The listing builds one solid part. Answer for the finished solid, in the listing's coordinates (mm). Coordinates: 2 decimals unless noted, no trailing zeros. Loops run counter-clockwise (first coordinate to the right, second up) from the corner with the lowest first, then second, coordinate; pieces in that order, holes last. Notation, with made-up numbers: (18.25, -6) -> (70.25, -6) arc R8 ccw to (70.25, 8) -> close; hole circle Ø4 at (20, 61.25). An arc over 180 degrees is marked (long way). Answer in a Markdown table with one row per item.
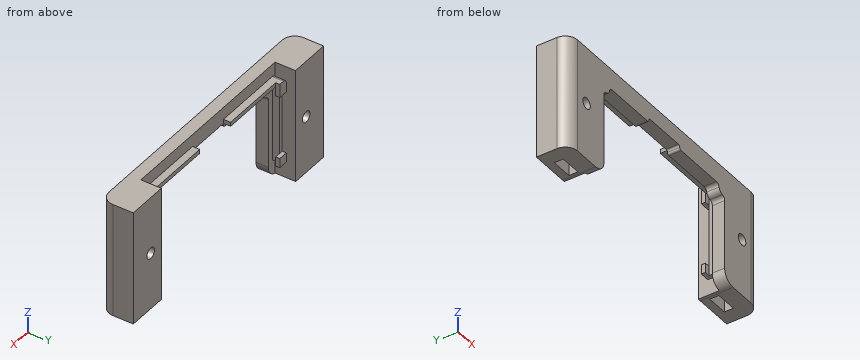
```python
from build123d import *

# Parameters (mm, degrees)
SKETCH1_R                = 8.05
SKETCH1_R_2              = 0.8
BOSS_EXTRUDE1_DEPTH      = 3
SKETCH1_5_R              = 0.8
BOSS_EXTRUDE3_DEPTH      = 3
CUT_EXTRUDE2_REACH       = 32.121
SKETCH5_R                = 8.05
FILLET2_R                = 1
BOSS_EXTRUDE4_DEPTH      = 1.75
BOSS_EXTRUDE7_START      = 1.75
SKETCH6_5_W              = 2.32
SKETCH6_5_H              = 2.32
BOSS_EXTRUDE7_DEPTH      = 1
SKETCH7_W                = 10
SKETCH7_H                = 28
BOSS_EXTRUDE8_DEPTH      = 8
SKETCH8_R                = 1.35
CUT_EXTRUDE3_DEPTH       = 1.1
CUT_EXTRUDE4_DEPTH       = 38.01634774
CUT_EXTRUDE4_DEPTH_BACK  = 38.01634774
SKETCH8_3_R              = 1.35
BOSS_EXTRUDE9_DEPTH      = 20
BOSS_EXTRUDE9_DEPTH_BACK = 20
SKETCH10_W               = 5
SKETCH10_H               = 3
CUT_EXTRUDE5_REACH       = 39.539
SKETCH9_W                = 43
SKETCH9_H                = 7.971706725
CUT_EXTRUDE6_REACH       = 39.016
SKETCH12_W               = 11
SKETCH12_H               = 1
FILLET3_R                = 3
FILLET4_START            = -1
FILLET4_DEPTH            = 5
FILLET4_2_DEPTH          = 3


with BuildPart() as part:
    # Sketch1 → Boss-Extrude1 (new body)
    with BuildSketch(Plane(origin=(0, 0, 0), x_dir=(1, 0, 0), z_dir=(0, 1, 0))):
        with BuildLine():
            Line((5.5, -7), (5.5, -14))
            Line((5.5, -14), (25.5, -14))
            ThreePointArc((25.5, -14), (26.207106781, -13.707106781), (26.5, -13))
            Line((26.5, -13), (26.5, 13))
            ThreePointArc((26.5, 13), (26.207106781, 13.707106781), (25.5, 14))
            Line((25.5, 14), (-25.5, 14))
            ThreePointArc((-25.5, 14), (-26.207106781, 13.707106781), (-26.5, 13))
            Line((-26.5, 13), (-26.5, -13))
            ThreePointArc((-26.5, -13), (-26.207106781, -13.707106781), (-25.5, -14))
            Line((-25.5, -14), (-5.5, -14))
            Line((-5.5, -14), (-5.5, -7))
            Line((-5.5, -7), (5.5, -7))
        make_face()
        with Locations(Location((-12.95, 0, 0), (0, 0, 270))):
            Circle(SKETCH1_R, mode=Mode.SUBTRACT)
        with Locations(Location((12.95, 0, 0), (0, 0, 270))):
            Circle(SKETCH1_R, mode=Mode.SUBTRACT)
        with BuildLine():
            ThreePointArc((-3.25, 5.75), (-5.25, 7.75), (-3.25, 9.75))
            Line((-3.25, 9.75), (3.25, 9.75))
            ThreePointArc((3.25, 9.75), (5.25, 7.75), (3.25, 5.75))
            Line((3.25, 5.75), (-3.25, 5.75))
        make_face(mode=Mode.SUBTRACT)
        with Locations(Location((-20.99, 8.49, 0), (0, 0, 270))):
            Circle(SKETCH1_R_2, mode=Mode.SUBTRACT)
        with Locations(Location((20.99, 8.49, 0), (0, 0, 270))):
            Circle(SKETCH1_R_2, mode=Mode.SUBTRACT)
        with Locations(Location((20.99, -8.49, 0), (0, 0, 270))):
            Circle(SKETCH1_R_2, mode=Mode.SUBTRACT)
        with Locations(Location((-20.99, -8.49, 0), (0, 0, 270))):
            Circle(SKETCH1_R_2, mode=Mode.SUBTRACT)
    extrude(amount=BOSS_EXTRUDE1_DEPTH)

    # Sketch1<5> → Boss-Extrude3 (add)
    with BuildSketch(Plane(origin=(0, 0, 0), x_dir=(1, 0, 0), z_dir=(0, 1, 0))):
        with Locations((20.99, 8.49)):
            Circle(SKETCH1_5_R)
        with Locations((-20.99, 8.49)):
            Circle(SKETCH1_5_R)
        with Locations((-20.99, -8.49)):
            Circle(SKETCH1_5_R)
        with Locations((20.99, -8.49)):
            Circle(SKETCH1_5_R)
    extrude(amount=BOSS_EXTRUDE3_DEPTH)

    # Sketch5 → Cut-Extrude2 (cut, up to next)
    with BuildSketch(Plane(origin=(0, 3, 0), x_dir=(1, 0, 0), z_dir=(0, 1, 0)), mode=Mode.PRIVATE) as cut_extrude2_sk1:
        with BuildLine():
            Line((3.25, 5.75), (-3.25, 5.75))
            ThreePointArc((-3.25, 5.75), (-5.052775638, 6.883974596), (-4.8112495, 9))
            Line((-4.8112495, 9), (-19.56873296, 9))
            ThreePointArc((-19.56873296, 9), (-19.502348624, 8.748830803), (-19.48, 8.49))
            ThreePointArc((-19.48, 8.49), (-20.12109264, 7.255050608), (-21.5, 7.06873296))
            Line((-21.5, 7.06873296), (-21.5, -7.06873296))
            ThreePointArc((-21.5, -7.06873296), (-20.12109264, -7.255050608), (-19.48, -8.49))
            ThreePointArc((-19.48, -8.49), (-19.502348624, -8.748830803), (-19.56873296, -9))
            Line((-19.56873296, -9), (-5.5, -9))
            Line((-5.5, -9), (-5.5, -7))
            Line((-5.5, -7), (5.5, -7))
            Line((5.5, -7), (5.5, -9))
            Line((5.5, -9), (19.56873296, -9))
            ThreePointArc((19.56873296, -9), (19.92226876, -7.42226876), (21.5, -7.06873296))
            Line((21.5, -7.06873296), (21.5, 7.06873296))
            ThreePointArc((21.5, 7.06873296), (19.92226876, 7.42226876), (19.56873296, 9))
            Line((19.56873296, 9), (4.8112495, 9))
            ThreePointArc((4.8112495, 9), (5.052775638, 6.883974596), (3.25, 5.75))
        make_face()
        with Locations((-12.95, 0)):
            Circle(SKETCH5_R, mode=Mode.SUBTRACT)
        with Locations((12.95, 0)):
            Circle(SKETCH5_R, mode=Mode.SUBTRACT)
    cut_extrude2_tool1 = extrude(cut_extrude2_sk1.sketch, amount=-CUT_EXTRUDE2_REACH, mode=Mode.PRIVATE) & part.part
    add(cut_extrude2_tool1.solids().sort_by_distance((0, 3, 0.207713))[0], mode=Mode.SUBTRACT)

    # Fillet2
    fillet2_edges = [part.edges().sort_by_distance(p)[0] for p in [
        (21.5, 1.5, 7.06873296),
        (19.56873296, 1.5, 9),
        (5.5, 1.5, 9),
        (-5.5, 1.5, 9),
        (-19.56873296, 1.5, 9),
        (-21.5, 1.5, 7.06873296),
        (-21.5, 1.5, -7.06873296),
        (-19.56873296, 1.5, -9),
        (-4.8112495, 1.5, -9),
        (4.8112495, 1.5, -9),
        (19.56873296, 1.5, -9),
        (21.5, 1.5, -7.06873296),
    ]]
    fillet(fillet2_edges, radius=FILLET2_R)

    # Sketch6 → Boss-Extrude4 (add)
    with BuildSketch(Plane(origin=(0, 3, 0), x_dir=(1, 0, 0), z_dir=(0, 1, 0))):
        with BuildLine():
            ThreePointArc((-23.9, -10), (-23.607106781, -10.707106781), (-22.9, -11))
            Line((-22.9, -11), (-5.5, -11))
            Line((-5.5, -11), (-5.5, -10))
            Line((-5.5, -10), (-22.9, -10))
            Line((-22.9, -10), (-22.9, 10))
            Line((-22.9, 10), (-23.9, 10))
            Line((-23.9, 10), (-23.9, -10))
        make_face()
    boss_extrude4 = extrude(amount=BOSS_EXTRUDE4_DEPTH)

    # Sketch6<5> → Boss-Extrude7 (add)
    with BuildSketch(Plane(origin=(0, 3, 0), x_dir=(1, 0, 0), z_dir=(0, 1, 0)).offset(BOSS_EXTRUDE7_START)):
        with BuildLine():
            Line((-23.9, -7.68), (-23.9, -10))
            ThreePointArc((-23.9, -10), (-23.607106781, -10.707106781), (-22.9, -11))
            Line((-22.9, -11), (-21.58, -11))
            Line((-21.58, -11), (-21.58, -7.68))
            Line((-21.58, -7.68), (-23.9, -7.68))
        make_face()
        with Locations((-22.74, 8.84)):
            Rectangle(SKETCH6_5_W, SKETCH6_5_H)
    boss_extrude7 = extrude(amount=BOSS_EXTRUDE7_DEPTH)

    # Mirror1: Boss-Extrude4, Boss-Extrude7 across plane
    add(boss_extrude4.mirror(Plane(origin=(0, 0, 0), x_dir=(0, 0, 1), z_dir=(1, 0, 0))))
    add(boss_extrude7.mirror(Plane(origin=(0, 0, 0), x_dir=(0, 0, 1), z_dir=(1, 0, 0))))

    # Sketch7 → Boss-Extrude8 (add)
    with BuildSketch(Plane(origin=(0, 0, 0), x_dir=(1, 0, 0), z_dir=(0, 1, 0))):
        with Locations((-28.9, 0)):
            Rectangle(SKETCH7_W, SKETCH7_H)
        with Locations((28.9, 0)):
            Rectangle(SKETCH7_W, SKETCH7_H)
    extrude(amount=BOSS_EXTRUDE8_DEPTH)

    # Sketch8 → Cut-Extrude3 (cut, symmetric)
    with BuildSketch(Plane(origin=(0, 5, 0), x_dir=(-1, 0, 0), z_dir=(0, -1, 0))):
        Polygon((-30.3, 1.5011107), (-30.3, -1.5011107), (-27.7, -3.0022214), (-25.1, -1.5011107), (-25.1, 1.5011107), (-27.7, 3.0022214), align=None)
        Polygon((-25.1, 1.5011107), (-25.1, 14), (-30.3, 14), (-30.3, 1.5011107), (-27.7, 3.0022214), align=None)
        Polygon((25.1, 14), (30.3, 14), (30.3, 1.5011107), (27.7, 3.0022214), (25.1, 1.5011107), align=None)
        Polygon((30.3, -1.5011107), (27.7, -3.0022214), (25.1, -1.5011107), (25.1, 1.5011107), (27.7, 3.0022214), (30.3, 1.5011107), align=None)
        with Locations((27.7, 0)):
            Circle(SKETCH8_R)
        with Locations((-27.7, 0)):
            Circle(SKETCH8_R)
    extrude(amount=CUT_EXTRUDE3_DEPTH, both=True, mode=Mode.SUBTRACT)

    # Sketch8<3> → Cut-Extrude4 (cut, two sides: drawn at the far end of the back side and taken through both)
    with BuildSketch(Plane(origin=(0, 5, 0), x_dir=(-1, 0, 0), z_dir=(0, -1, 0)).offset(-CUT_EXTRUDE4_DEPTH_BACK)):
        with Locations(Location((-27.7, 0, 0), (0, 0, 90))):
            Circle(SKETCH8_3_R)
        with Locations(Location((27.7, 0, 0), (0, 0, 90))):
            Circle(SKETCH8_3_R)
    extrude(amount=CUT_EXTRUDE4_DEPTH + CUT_EXTRUDE4_DEPTH_BACK, mode=Mode.SUBTRACT)

    # Sketch10 → Boss-Extrude9 (add, two sides: drawn at the far end of the back side and taken through both)
    with BuildSketch(Plane(origin=(-5.5, 0, 0), x_dir=(0, 0, -1), z_dir=(1, 0, 0)).offset(-BOSS_EXTRUDE9_DEPTH_BACK)):
        with Locations((-11.5, 1.5)):
            Rectangle(SKETCH10_W, SKETCH10_H)
    extrude(amount=BOSS_EXTRUDE9_DEPTH + BOSS_EXTRUDE9_DEPTH_BACK)

    # Sketch9 → Cut-Extrude5 (cut, up to next)
    with BuildSketch(Plane.XZ, mode=Mode.PRIVATE) as cut_extrude5_sk1:
        with Locations((0, -10.014146637)):
            Rectangle(SKETCH9_W, SKETCH9_H)
    cut_extrude5_tool1 = extrude(cut_extrude5_sk1.sketch, amount=-CUT_EXTRUDE5_REACH, mode=Mode.PRIVATE) & part.part
    add(cut_extrude5_tool1.solids().sort_by_distance((0, 0, -10.014147))[0], mode=Mode.SUBTRACT)

    # Sketch12 → Cut-Extrude6 (cut, up to next)
    with BuildSketch(Plane(origin=(0, 3, 0), x_dir=(1, 0, 0), z_dir=(0, 1, 0)), mode=Mode.PRIVATE) as cut_extrude6_sk1:
        with Locations((0, -9.5)):
            Rectangle(SKETCH12_W, SKETCH12_H)
    cut_extrude6_tool1 = extrude(cut_extrude6_sk1.sketch, amount=-CUT_EXTRUDE6_REACH, mode=Mode.PRIVATE) & part.part
    add(cut_extrude6_tool1.solids().sort_by_distance((0, 3, 9.5))[0], mode=Mode.SUBTRACT)

    # Fillet3
    fillet3_edges = [part.edges().sort_by_distance(p)[0] for p in [
        (33.9, 0, 0),
        (-33.9, 0, 0),
        (21.5, 1.5, -14),
        (-21.5, 1.5, -14),
    ]]
    fillet(fillet3_edges, radius=FILLET3_R)

    # Fillet4: read off the stored shape, not the designer's step
    # Fillet4 outline → Fillet4 (cut)
    with BuildSketch(Plane(origin=(0, 0, 0), x_dir=(1, 0, 0), z_dir=(0, 1, 0)).offset(FILLET4_START)):
        with BuildLine():
            Line((5.5, -9), (5.5, -9.5))
            ThreePointArc((5.5, -9.5), (5.646446609, -9.146446609), (6, -9))
            Line((6, -9), (5.5, -9))
        make_face()
        with BuildLine():
            ThreePointArc((-6, -9), (-5.646446609, -9.146446609), (-5.5, -9.5))
            Line((-5.5, -9.5), (-5.5, -9))
            Line((-5.5, -9), (-6, -9))
        make_face()
    extrude(amount=FILLET4_DEPTH, mode=Mode.SUBTRACT)

    # Fillet4 2 outline → Fillet4 2 (add)
    with BuildSketch(Plane(origin=(0, 0, 0), x_dir=(1, 0, 0), z_dir=(0, 1, 0))):
        with BuildLine():
            ThreePointArc((5.5, -9.5), (5.353553391, -9.853553391), (5, -10))
            Line((5, -10), (5.5, -10))
            Line((5.5, -10), (5.5, -9.5))
        make_face()
        with BuildLine():
            ThreePointArc((-5, -10), (-5.353553391, -9.853553391), (-5.5, -9.5))
            Line((-5.5, -9.5), (-5.5, -10))
            Line((-5.5, -10), (-5, -10))
        make_face()
    extrude(amount=FILLET4_2_DEPTH)


solid = part.part
```
Item 1: A cutting plane is placed at B-B, the plane y = 6.75. Determine the outline of the cut face in (x, z).
Findings below:
| item | result |
|---|---|
| outline | (-33.9, -14) -> (-24.5, -14) arc R3 ccw to (-23.9, -13.94) -> (-23.9, 14) -> (-33.9, 14) -> close; (23.9, -13.94) arc R3 ccw to (24.5, -14) -> (33.9, -14) -> (33.9, 14) -> (23.9, 14) -> close; hole circle Ø2.7 at (-27.7, 0); hole circle Ø2.7 at (27.7, 0) |
Item 2: A cutting plane is placed at A-A, the plane z = -3.5. Determine the outline of the cut face in (x, y).
Findings below:
| item | result |
|---|---|
| outline | (-33.9, 3) arc R3 ccw to (-30.9, 0) -> (-21.5, 0) -> (-21.5, 3) -> (-22.9, 3) -> (-22.9, 4.75) -> (-23.9, 4.75) -> (-23.9, 8) -> (-33.9, 8) -> close; (21.5, 0) -> (30.9, 0) arc R3 ccw to (33.9, 3) -> (33.9, 8) -> (23.9, 8) -> (23.9, 4.75) -> (22.9, 4.75) -> (22.9, 3) -> (21.5, 3) -> close; hole (-30.3, 3.9) -> (-25.1, 3.9) -> (-25.1, 6.1) -> (-30.3, 6.1) -> close; hole (25.1, 3.9) -> (30.3, 3.9) -> (30.3, 6.1) -> (25.1, 6.1) -> close |
Item 3: Flat-ended cylindrical pins translate along their axes: pin 1 Ø0.9 at (x, y) = (-13.5, 2) entering from -Z; pin 2 Ø1 at (x, y) = (-5.5, 6.5) entering from -Z; pin 3 Ø1 at (x, y) = (9, 4) entering from -Z; pin 4 Ø1.5 at (y, z) = (2, -6.5) entering from +X. Find the tip coordinate at first contact, or state that the pin passes through.
Findings below:
| item | result |
|---|---|
| pin 1 | stops at z = 9 |
| pin 2 | passes through |
| pin 3 | stops at z = 10 |
| pin 4 | stops at x = 33.89 |
Item 4: A cutting plane is placed at D-D, the plane x = -12.5. Determine the outline of the cut face in (y, z).
Findings below:
| item | result |
|---|---|
| outline | (0, 9) -> (3, 9) -> (3, 10) -> (4.75, 10) -> (4.75, 11) -> (3, 11) -> (3, 14) -> (0, 14) -> close |
Item 5: A cutting plane is placed at C-C, the plane z = 12.25. Determine the outline of the cut face in (x, y), plus the area to 3 significant figures.
Findings below:
| item | result |
|---|---|
| outline | (-33.9, 3) arc R3 ccw to (-30.9, 0) -> (30.9, 0) arc R3 ccw to (33.9, 3) -> (33.9, 8) -> (23.9, 8) -> (23.9, 3) -> (-23.9, 3) -> (-23.9, 8) -> (-33.9, 8) -> close |
| area | 300 mm2 |
Item 6: Find the intervals of material crossed by probe 1 along X at (y, z) = (7, 0); probe 2 along X at (y, z) = (4, -7); probe 3 along X at (y, z) = (6.5, -10.25), in increasing order.
Findings below:
| item | result |
|---|---|
| probe 1 | x = -33.9 to -29.05, -26.35 to -23.9, 23.9 to 26.35, 29.05 to 33.9 |
| probe 2 | x = -33.9 to -30.3, -25.1 to -22.9, 22.9 to 25.1, 30.3 to 33.9 |
| probe 3 | x = -33.9 to -23.9, 23.9 to 33.9 |
